from build123d import *

# Parameters (mm, degrees)
F0_R     = 15
F0_R_2   = 10
F1_DEPTH = 200
F3_W     = 572.0791816711
F3_H     = 457.3649317026
F3_R     = 100
F4_DEPTH = 60
F6_R     = 95
F7_DEPTH = 5
F6_R_2   = 100
F8_DEPTH = 200
F9_D     = 20
F9_DEPTH = 200.0010001


with BuildPart() as f1:
    # F0 (on Front) → F1 (new body)
    with BuildSketch(Plane.XZ):
        with Locations((-85, 15)):
            Circle(F0_R)
        with Locations((-85, 15)):
            Circle(F0_R_2, mode=Mode.SUBTRACT)
    extrude(amount=F1_DEPTH)

    # F3 (on offset) → F4 (intersect)
    with BuildSketch(Plane.XY.offset(-20)):
        with Locations((-14.546662569, -7.4936076999)):
            Rectangle(F3_W, F3_H)
        Circle(F3_R, mode=Mode.SUBTRACT)
    extrude(amount=F4_DEPTH, mode=Mode.INTERSECT)



with BuildPart() as f7:
    # F6 (on Top) → F7 (new body)
    with BuildSketch(Plane.XY):
        Circle(F6_R)
    extrude(amount=F7_DEPTH)


with BuildPart() as f1_1:
    add(f1.part)

    add(f7.part)  # F8 merges F7
    # F6 (on Top) → F8 (join)
    with BuildSketch(Plane.XY):
        Circle(F6_R_2)
        Circle(F6_R, mode=Mode.SUBTRACT)
    extrude(amount=F8_DEPTH)

    # F9 (through all, one way)
    with BuildSketch(Plane(origin=(0, 0, 0), x_dir=(1, 0, 0), z_dir=(0, 1, 0))):
        with Locations((-85, -15)):
            Circle(F9_D / 2)
    extrude(amount=-F9_DEPTH, mode=Mode.SUBTRACT)


solid = f1_1.part
The listing builds one solid part. Answer for the finished solid, in the listing's coordinates (mm). A direction names the side the tool comes from. Give positions to 0.01 mm unless a question says otherwise; leave off trailing zeros. Loops run counter-clockwise (first coordinate to the right, second up) from the corner with the lowest first, then second, coordinate; pieces in that order, holes last. Notation, with made-up numbers: M -34.75,-29 L 24.25,-29 A28 ccw 24.25,2 Z; hole C 28,-13.75 d5. An arc over 180 degrees is marked long. Answer as CSV lines item,"result".
Item 1: Given pin 1 Ø5 at (x, z) = (23, 95.5) entering from +Y; pin 2 Ø6 at (x, y) = (22.5, -43.5) entering from +Z; pin 3 Ø2 at (x, z) = (-78.5, 130.5) entering from +Y, each flat-ended and moving along its own axis, determine where each tip first touches the part or whether it passes through.
Values follow:
pin 1,"stops at y = 97.88"
pin 2,"stops at z = 5"
pin 3,"stops at y = 63.2"
Item 2: The part is cut by section C-C (y = -180.5). Give the vertices of the cut face in (x, z).
Values follow:
outline,"C -85,15 d30; hole C -85,15 d20"
Item 3: Which of the six approach directions +Z, -Z, +X, -X, +Y, -Y give full straight-line access (tool end or side, diameter ignored) to faces 1 (the flat face through (-1, 1, 5)), 2 (the flat face through (-75, -200, 12)), 3 (the cylindrical face through (-99.985, -120.822, 15.66))?
Values follow:
face 1,"+Z"
face 2,"+Z, -Z, +X, -X, -Y"
face 3,"-Y"
Item 4: The mould has two halves that part along X. Classify faces 4 (the flat face through (-1, 1, 0)), 5 (the cylindrical face through (90.61, 28.54, 101.13)): released by +X, released by -X, zero draft, split by the parting line, or undercut.
Values follow:
face 4,"zero draft"
face 5,"undercut"
Item 5: The part is cut by section B-B (z = 131). Give the vertices of the cut face in (x, y).
Values follow:
outline,"C 0,0 d200; hole C 0,0 d190"
Item 6: The part is cut by section D-D (z = 15). Give the vertices of the cut face in (x, y), and give its area (3 significant figures).
Values follow:
outline,"M -100,-200 L -95,-200 L -95,0 A95 cw long -75,-58.31 L -75,-200 L -70,-200 L -70,-71.41 A100 ccw long -100,0 Z"
area,"4,380 mm^2"
Item 7: The part is cut by section A-A (x = 0). Give the vertices of the cut face in (y, z), and give its area (3 significant figures).
Values follow:
outline,"M -100,0 L 100,0 L 100,200 L 95,200 L 95,5 L -95,5 L -95,200 L -100,200 Z"
area,"2,950 mm^2"
Item 8: Straight lines are drawn through the part: line 1 along Z through (x, y) = (-85, -165.5); line 2 along X through (y, z) = (-59, 134.5); line 3 along Y through (x, z) = (56.5, 97). For each, find the intervals that lie inside material, in ascending order. Write a range as [from, to].
Values follow:
line 1,"z = [0, 5], [25, 30]"
line 2,"x = [-80.74, -74.46], [74.46, 80.74]"
line 3,"y = [-82.51, -76.37], [76.37, 82.51]"
